Part model, mm, in its own coordinate system. Round coordinates to 2 decimals unless told otherwise and drop trailing zeros. Order: outer loops, then holes, each group sorted by start corner. A loop starts at its lowest first (then second) coordinate and runs counter-clockwise, first axis right, second up. Notation, with made-up numbers: (38.25, 60) - (91.25, 60) arc R20 cw to (91.25, 90) - close; hole circle Ø8 at (77, -3.75). An arc over 180 degrees is marked (long way). Return JSON: item names as keys, results as strings. Group by question number.
Item 1: Saw through at B-B on z = 296. List the corners of the cut face in (x, y), and give its area (3 significant figures).
Item 2: Saw through at C-C on y = -83.5. List the corners of the cut face in (x, z).
Item 3: Saw through at A-A on z = 231.5. List the corners of the cut face in (x, y), and give its area (3 significant figures).
Item 4: Drop flat-ended pins along their axis: pin 1 (1 mm diameter, centred on y = -124, z = 51, fed in from +X); pin 2 (12 mm diameter, centred on x = -129.5, z = 176, fed in from -Y); pin 3 (6 mm diameter, centred on x = -91.5, z = 102.5, fed in from +Y). Give the stop position or say it passes through.
Item 5: Probe probe 1 along X at (y, z) = (-182.5, 226); probe 2 along Y at (x, z) = (-134, 128); probe 3 along X at (y, z) = (-62, 268). List the from-to ranges inside material, lowest first.
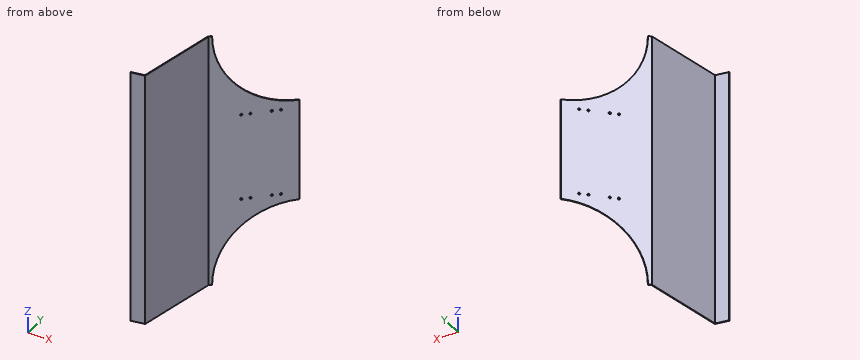
```python
from build123d import *

# Parameters (mm, degrees)
EXTRUDE_1_DEPTH     = 380
SKETCH_2_R          = 1.5
CUT_EXTRUDE_1_DEPTH = 3


with BuildPart() as part:
    # 草图1 → 凸台-拉伸1 (new body)
    with BuildSketch(Plane.XY):
        Polygon((-133.074926411, -194.523734135), (-152.081511659, -197.875107926), (-151.907863481, -198.859915679), (-132.211708421, -195.386952125), (-111.394108644, -77.324476981), (-27.25197302, 6.817658643), (-27.959079801, 7.524765424), (-112.324165337, -76.840320111), align=None)
    extrude(amount=EXTRUDE_1_DEPTH)

    # 草图2 → 切除-拉伸1 (cut)
    with BuildSketch(Plane(origin=(-17.034815832, 17.034815832, 0), x_dir=(0, 0, -1), z_dir=(0.7071067811865477, -0.7071067811865475, 0))):
        with Locations(Location((-254.5, -38.449242265, 0), (0, 0, 90))):
            Circle(SKETCH_2_R)
        with Locations(Location((-254.5, -50.449242265, 0), (0, 0, 90))):
            Circle(SKETCH_2_R)
        with BuildLine():
            ThreePointArc((-380, -128.449242265), (-299.389826945, -95.05941532), (-266, -14.449242265))
            Line((-266, -14.449242265), (-380, -14.449242265))
            Line((-380, -14.449242265), (-380, -128.449242265))
        make_face()
        with BuildLine():
            Line((-380, -14.449242265), (-266, -14.449242265))
            ThreePointArc((-266, -14.449242265), (-460.610173055, 66.16093079), (-380, -128.449242265))
            Line((-380, -128.449242265), (-380, -14.449242265))
        make_face()
        with BuildLine():
            ThreePointArc((114, -14.449242265), (0, 99.550757735), (-114, -14.449242265))
            Line((-114, -14.449242265), (0, -14.449242265))
            Line((0, -14.449242265), (0, -128.449242265))
            ThreePointArc((0, -128.449242265), (80.610173055, -95.05941532), (114, -14.449242265))
        make_face()
        with BuildLine():
            Line((0, -14.449242265), (-114, -14.449242265))
            ThreePointArc((-114, -14.449242265), (-80.610173055, -95.05941532), (0, -128.449242265))
            Line((0, -128.449242265), (0, -14.449242265))
        make_face()
        with Locations(Location((-125.5, -38.449242265, 0), (0, 0, 90))):
            Circle(SKETCH_2_R)
        with Locations(Location((-125.5, -50.449242265, 0), (0, 0, 90))):
            Circle(SKETCH_2_R)
        with Locations(Location((-125.5, -78.449242265, 0), (0, 0, 90))):
            Circle(SKETCH_2_R)
        with Locations(Location((-125.5, -90.449242265, 0), (0, 0, 90))):
            Circle(SKETCH_2_R)
        with Locations(Location((-254.5, -90.449242265, 0), (0, 0, 90))):
            Circle(SKETCH_2_R)
        with Locations(Location((-254.5, -78.449242265, 0), (0, 0, 90))):
            Circle(SKETCH_2_R)
    extrude(amount=-CUT_EXTRUDE_1_DEPTH, mode=Mode.SUBTRACT)


solid = part.part
```
Filled in:
{
 "1": {"outline": "(-152.08, -197.88) - (-151.91, -198.86) - (-132.21, -195.39) - (-111.39, -77.32) - (-81.75, -47.68) - (-82.46, -46.97) - (-112.32, -76.84) - (-133.07, -194.52) - close", "area": "181 mm^2"},
 "2": {"outline": "(-113.5, 0) - (-112.48, 0) - (-112.48, 380) - (-113.5, 380) - close"},
 "3": {"outline": "(-152.08, -197.88) - (-151.91, -198.86) - (-132.21, -195.39) - (-111.39, -77.32) - (-27.25, 6.82) - (-27.96, 7.52) - (-112.32, -76.84) - (-133.07, -194.52) - close", "area": "258 mm^2"},
 "4": {"pin 1": "stops at x = -119.54", "pin 2": "stops at y = -195.97", "pin 3": "stops at y = -53.02"},
 "5": {"probe 1": "x = -130.95 to -129.94", "probe 2": "y = -195.7 to -194.69", "probe 3": "x = -97.48 to -96.07"}
}
